from build123d import *

# Parameters (mm, degrees)
SKETCH1_W           = 31.75
SKETCH1_H           = 38.1
SKETCH1_R           = 7.1374
SKETCH1_R_2         = 1.2
SKETCH1_R_3         = 1.905
BOSS_EXTRUDE1_DEPTH = 1.5875
BOSS_EXTRUDE3_DEPTH = 1.5875
CUT_EXTRUDE1_DEPTH  = 2.5875
FILLET3_R           = 2.54
FILLET2_R           = 2.286


with BuildPart() as part:
    # Sketch1 → Boss-Extrude1 (new body)
    with BuildSketch(Plane(origin=(0, 0, 0), x_dir=(1, 0, 0), z_dir=(0, 1, 0))):
        Rectangle(SKETCH1_W, SKETCH1_H)
        Circle(SKETCH1_R, mode=Mode.SUBTRACT)
        with Locations((-6.363961031, -6.363961031)):
            Circle(SKETCH1_R_2, mode=Mode.SUBTRACT)
        with Locations((-6.363961031, 6.363961031)):
            Circle(SKETCH1_R_2, mode=Mode.SUBTRACT)
        with Locations((6.363961031, 6.363961031)):
            Circle(SKETCH1_R_2, mode=Mode.SUBTRACT)
        with Locations((6.363961031, -6.363961031)):
            Circle(SKETCH1_R_2, mode=Mode.SUBTRACT)
        with Locations((-12.065, -15.24)):
            Circle(SKETCH1_R_3, mode=Mode.SUBTRACT)
        with Locations((-12.065, 15.24)):
            Circle(SKETCH1_R_3, mode=Mode.SUBTRACT)
        with Locations((12.065, 15.24)):
            Circle(SKETCH1_R_3, mode=Mode.SUBTRACT)
        with Locations((12.065, -15.24)):
            Circle(SKETCH1_R_3, mode=Mode.SUBTRACT)
    extrude(amount=BOSS_EXTRUDE1_DEPTH)

    # Sketch3 → Boss-Extrude3 (add, through all)
    with BuildSketch(Plane(origin=(0, 1.5875, 0), x_dir=(1, 0, 0), z_dir=(0, 1, 0))):
        with BuildLine():
            Line((-3.258830889, 6.35), (3.258830889, 6.35))
            ThreePointArc((3.258830889, 6.35), (0, 7.1374), (-3.258830889, 6.35))
        make_face()
        with BuildLine():
            Line((3.258830889, -6.35), (-3.258830889, -6.35))
            ThreePointArc((-3.258830889, -6.35), (0, -7.1374), (3.258830889, -6.35))
        make_face()
    extrude(amount=-BOSS_EXTRUDE3_DEPTH)

    # Sketch4 → Cut-Extrude1 (cut, through all)
    with BuildSketch(Plane.XZ):
        with BuildLine():
            Line((-15.875, 14.296387236), (-15.875, -14.296387236))
            ThreePointArc((-15.875, -14.296387236), (-12.2174, 0), (-15.875, 14.296387236))
        make_face()
        with BuildLine():
            Line((15.875, -14.296387236), (15.875, 14.296387236))
            ThreePointArc((15.875, 14.296387236), (12.2174, 0), (15.875, -14.296387236))
        make_face()
    extrude(amount=-CUT_EXTRUDE1_DEPTH, mode=Mode.SUBTRACT)

    # Fillet3
    fillet3_edges = [part.edges().sort_by_distance(p)[0] for p in [
        (-15.875, 0.79375, 14.296387236),
        (-15.875, 0.79375, -14.296387236),
        (15.875, 0.79375, 19.05),
        (-15.875, 0.79375, 19.05),
        (15.875, 0.79375, -14.296387236),
        (-15.875, 0.79375, -19.05),
        (15.875, 0.79375, 14.296387236),
        (15.875, 0.79375, -19.05),
    ]]
    fillet(fillet3_edges, radius=FILLET3_R)

    # Fillet2
    fillet2_edges = [part.edges().sort_by_distance(p)[0] for p in [
        (-3.258830889, 0.79375, -6.35),
        (3.258830889, 0.79375, -6.35),
        (3.258830889, 0.79375, 6.35),
        (-3.258830889, 0.79375, 6.35),
    ]]
    fillet(fillet2_edges, radius=FILLET2_R)


solid = part.part
Can you work these out from the model? Positions are in its coordinate system, mm. A direction names the side the tool comes from. Give positions to 0.01 mm unless a question says otherwise; leave off trailing zeros. Loops run counter-clockwise (first coordinate to the right, second up) from the corner with the lowest first, then second, coordinate; pieces in that order, holes last. Notation, with made-up numbers: (-38.75, 8.5) -> (4.25, 8.5) arc R17 ccw to (4.25, 29.5) -> close; hole circle Ø8 at (-40, -1.5). An arc over 180 degrees is marked (long way). Return JSON: item names as keys, results as strings.
Q1. I want a section at D-D, the plane y = 1.25. Count the separate pieces of the cut face and the enclosed holes in it, then the cut area to 3 significant figures.
Checks:
{"separate pieces": "1", "enclosed holes": "9", "area": "846 mm2"}
Q2. For pin 1 Ø1.9 at (x, z) = (6.36, 6.36) entering from +Y; pin 2 Ø6 at (x, z) = (-12.065, -15.24) entering from -Y, each with a flat end and sliding along its axis, tell me the tip position at first contact or that it passes through.
Checks:
{"pin 1": "passes through", "pin 2": "stops at y = 0"}
Q3. I want a section at C-C, the plane x = -11. List the corners of the cut face in (y, z) for me, then the cut area to 3 significant figures.
Checks:
{"outline": "(0, -19.05) -> (1.59, -19.05) -> (1.59, -16.82) -> (0, -16.82) -> close; (0, -13.66) -> (1.59, -13.66) -> (1.59, 13.66) -> (0, 13.66) -> close; (0, 16.82) -> (1.59, 16.82) -> (1.59, 19.05) -> (0, 19.05) -> close", "area": "50.5 mm2"}
Q4. I want a section at A-A, the plane x = -1. List the corners of the cut face in (y, z) for me, then the cut area to 3 significant figures.
Checks:
{"outline": "(0, -19.05) -> (1.59, -19.05) -> (1.59, -6.35) -> (0, -6.35) -> close; (0, 6.35) -> (1.59, 6.35) -> (1.59, 19.05) -> (0, 19.05) -> close", "area": "40.3 mm2"}
Q5. On a 3-axis mill with a long thin cutter (end or side, diameter ignored), from which of +Z, -Z, +X, -X, +Y, -Y can I reach the whole of each face in a straight line? I mean faces 1 (the face through (-15.8, 0.8, -14.32)), 2 (the face through (-7.137, 0.783, -0.099)), 3 (the face through (-15.151, 0.805, -18.286)). Say none if no direction works.
Checks:
{"face 1": "-X, +Y, -Y", "face 2": "+Y, -Y", "face 3": "-Z, -X, +Y, -Y"}
Q6. I need wall thicknesses on probe 1 along Z at (x, y) = (-12, 0.9); probe 2 along X at (y, z) = (1.1, 16) (3 decimals); probe 3 along Z at (x, y) = (6, 1.05). Which ranges of each line are inside material? Lowest first, please.
Checks:
{"probe 1": "z = -19.05 to -17.14, -13.34 to 13.34, 17.14 to 19.05", "probe 2": "x = -15.875 to -13.812, -10.318 to 10.318, 13.812 to 15.875", "probe 3": "z = -19.05 to -7.51, -5.22 to -3.87, 3.87 to 5.22, 7.51 to 19.05"}
Q7. I want a section at B-B, the plane z = -16. List the corners of the cut face in (x, y) for me (1 decimal), then the cut area to 3 significant figures.
Checks:
{"outline": "(-15.9, 0) -> (-13.8, 0) -> (-13.8, 1.6) -> (-15.9, 1.6) -> close; (-10.3, 0) -> (10.3, 0) -> (10.3, 1.6) -> (-10.3, 1.6) -> close; (13.8, 0) -> (15.9, 0) -> (15.9, 1.6) -> (13.8, 1.6) -> close", "area": "39.3 mm2"}
Q8. We'd pull the mould along Z, two halves only. Please class faces 4 (the face through (0, 1, -19.05)), 5 (the face through (10.553, 0.783, -14.081)), 6 (the face through (-7.3, 1.588, -0.3)): released by +Z, released by -Z, zero draft, split by the parting line, or undercut.
Checks:
{"face 4": "released by -Z", "face 5": "undercut", "face 6": "zero draft"}
